```python
from build123d import *

# Parameters (mm, degrees)
SKETCH_1_W          = 30
SKETCH_1_H          = 33
SKETCH_1_R          = 1.6
EXTRUDE_1_DEPTH     = 3
SKETCH_2_W          = 14.5
SKETCH_2_H          = 7
SKETCH_2_W_2        = 24
SKETCH_2_H_2        = 18.3
CUT_EXTRUDE_1_DEPTH = 4
FILLET_1_R          = 2
FILLET_2_R          = 2


with BuildPart() as part:
    # 草图1 → 凸台-拉伸1 (new body)
    with BuildSketch(Plane.XY):
        with Locations((15, 16.5)):
            Rectangle(SKETCH_1_W, SKETCH_1_H)
        with Locations((5, 31.3)):
            Circle(SKETCH_1_R, mode=Mode.SUBTRACT)
        with Locations((25, 31.3)):
            Circle(SKETCH_1_R, mode=Mode.SUBTRACT)
        with Locations((25, 2.6)):
            Circle(SKETCH_1_R, mode=Mode.SUBTRACT)
        with Locations((5, 2.6)):
            Circle(SKETCH_1_R, mode=Mode.SUBTRACT)
    extrude(amount=EXTRUDE_1_DEPTH)

    # 草图2 → 切除-拉伸1 (cut, through all)
    with BuildSketch(Plane.XY.offset(3)):
        with Locations((15, 3.5)):
            Rectangle(SKETCH_2_W, SKETCH_2_H)
        with Locations((15, 19.15)):
            Rectangle(SKETCH_2_W_2, SKETCH_2_H_2)
    extrude(amount=-CUT_EXTRUDE_1_DEPTH, mode=Mode.SUBTRACT)

    # 圆角1
    fillet_1_edges = [part.edges().sort_by_distance(p)[0] for p in [
        (0, 33, 1.5),
        (30, 33, 1.5),
        (30, 0, 1.5),
        (0, 0, 1.5),
    ]]
    fillet(fillet_1_edges, radius=FILLET_1_R)

    # 圆角2
    fillet_2_edges = [part.edges().sort_by_distance(p)[0] for p in [
        (7.75, 0, 1.5),
        (7.75, 7, 1.5),
        (22.25, 7, 1.5),
        (22.25, 0, 1.5),
        (3, 10, 1.5),
        (3, 28.3, 1.5),
        (27, 28.3, 1.5),
        (27, 10, 1.5),
    ]]
    fillet(fillet_2_edges, radius=FILLET_2_R)


solid = part.part
```
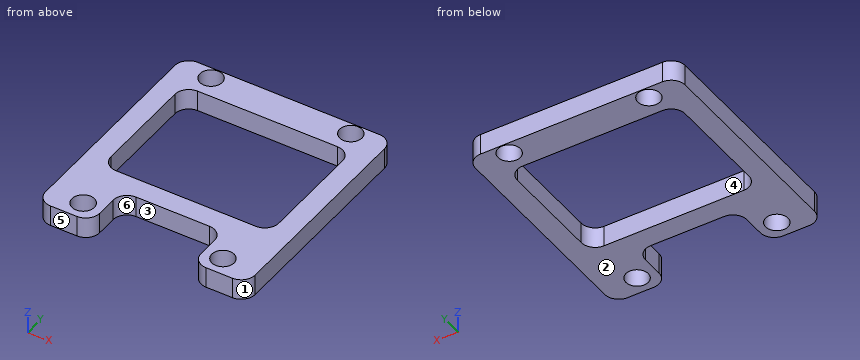
The model under review builds one solid part; all positions refer to its coordinate system, in mm. Face numbers are marked on the shaded views. A direction names the side the tool comes from. Round coordinates to 2 decimals unless told otherwise and drop trailing zeros. Loops run counter-clockwise (first coordinate to the right, second up) from the corner with the lowest first, then second, coordinate; pieces in that order, holes last.
1) Consider section C-C on z = 2.15. State the section outline as (x, y) points.
Values follow:
outline: (0, 2) arc R2 ccw to (2, 0) - (5.75, 0) arc R2 ccw to (7.75, 2) - (7.75, 5) arc R2 cw to (9.75, 7) - (20.25, 7) arc R2 cw to (22.25, 5) - (22.25, 2) arc R2 ccw to (24.25, 0) - (28, 0) arc R2 ccw to (30, 2) - (30, 31) arc R2 ccw to (28, 33) - (2, 33) arc R2 ccw to (0, 31) - close; hole (3, 12) arc R2 ccw to (5, 10) - (25, 10) arc R2 ccw to (27, 12) - (27, 26.3) arc R2 ccw to (25, 28.3) - (5, 28.3) arc R2 ccw to (3, 26.3) - close; hole circle Ø3.2 at (5, 2.6); hole circle Ø3.2 at (5, 31.3); hole circle Ø3.2 at (25, 2.6); hole circle Ø3.2 at (25, 31.3)
2) Tool access review of the marked faces 4, 5 and 6: name each direction out of +Z, -Z, +X, -X, +Y, -Y from which nothing blocks a thin tool from reaching the whole face with its end or side.
Values follow:
face 4: +Z, -Z
face 5: +Z, -Z, +X, -X, -Y
face 6: +Z, -Z, -Y
3) The part is to be moulded in two halves that separate along X. For the marked faces 1, 2 and 3, say which applies: pulls with the +X half, pulls with the -X half, needs draft (parallel to the pull), parting line crosses it, or undercut.
Values follow:
face 1: pulls with the +X half
face 2: needs draft
face 3: undercut
4) Wall thickness on line 1 along X through (y, z) = (24, 0.95); line 2 along Y through (x, z) = (10, 1.1); line 3 along X through (y, z) = (27.5, 1.9): over which ranges is each line inside the solid? List them lowest first.
Values follow:
line 1: x = 0 to 3, 27 to 30
line 2: y = 7 to 10, 28.3 to 33
line 3: x = 0 to 3.4, 26.6 to 30
5) Consider section D-D on y = 2.6. State the section outline as (x, z) points.
Values follow:
outline: (0, 0) - (3.4, 0) - (3.4, 3) - (0, 3) - close; (6.6, 0) - (7.75, 0) - (7.75, 3) - (6.6, 3) - close; (22.25, 0) - (23.4, 0) - (23.4, 3) - (22.25, 3) - close; (26.6, 0) - (30, 0) - (30, 3) - (26.6, 3) - close
6) Consider section B-B on x = 18. State the section outline as (y, z) points, then the cut area to 3 significant figures.
Values follow:
outline: (7, 0) - (10, 0) - (10, 3) - (7, 3) - close; (28.3, 0) - (33, 0) - (33, 3) - (28.3, 3) - close
area: 23.1 mm2
7) Consider section A-A on y = 16.5. State the section outline as (x, z) points, then the cut area to 3 significant figures.
Values follow:
outline: (0, 0) - (3, 0) - (3, 3) - (0, 3) - close; (27, 0) - (30, 0) - (30, 3) - (27, 3) - close
area: 18.0 mm2
